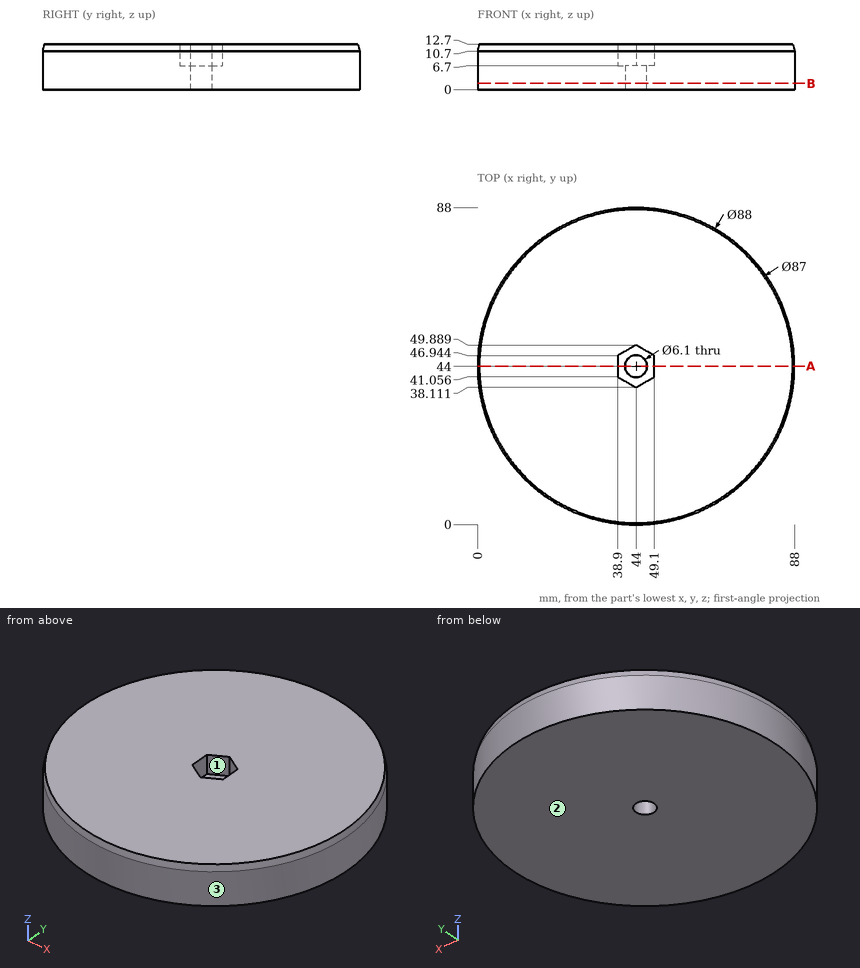
Study the drawing (mm; zero at the part's minimum x, y, z) and answer. Coordinates: 2 decimals unless noted, no trailing zeros. Loops run counter-clockwise (first coordinate to the right, second up) from the corner with the lowest first, then second, coordinate; pieces in that order, holes last. Notation, with made-up numbers: M 81,46.25 L 116,46.25 A13 cw 116,51.25 Z; hole C 45.25,22 d2. An arc over 180 degrees is marked long. Answer in a Markdown table with one row per item.
1) Find section B-B (z = 1.75). Determine the outline of the cut face in (x, y).
Answers below:
| item | result |
|---|---|
| outline | C 44,44 d88; hole C 44,44 d6.1 |
2) Find section A-A (y = 44). Determine the outline of the cut face in (x, z), then the cut area to 3 significant figures.
Answers below:
| item | result |
|---|---|
| outline | M 0,0 L 40.95,0 L 40.95,6.7 L 38.9,6.7 L 38.9,12.7 L 0.5,12.7 L 0,10.7 Z; M 47.05,0 L 88,0 L 88,10.7 L 87.5,12.7 L 49.1,12.7 L 49.1,6.7 L 47.05,6.7 Z |
| area | 1,010 mm^2 |
3) Determine the mould class of the marked faces 1, 2 and 3 for opening direction Y: released by +Y, released by -Y, zero draft, split by the parting line, or undercut.
Answers below:
| item | result |
|---|---|
| face 1 | undercut |
| face 2 | zero draft |
| face 3 | split by the parting line |
4) Given pin 1 (1.5 mm diameter, centred on x = 19, z = 4, fed in from +Y) (1 decimal); pin 2 (1 mm diameter, centred on x = 72.5, z = 10, fed in from +Y); pin 3 (5 mm diameter, centred on y = 55, z = 2.5, fed in from -X), each flat-ended and moving along its own axis, determine where each tip first touches the part or whether it passes through.
Answers below:
| item | result |
|---|---|
| pin 1 | y = 80.7 |
| pin 2 | y = 77.94 |
| pin 3 | x = 0.83 |
5) Find the intervals of material crossed by probe 1 along X at (y, z) = (44, 5.75); probe 2 along Z at (x, y) = (47.5, 47), in increasing order.
Answers below:
| item | result |
|---|---|
| probe 1 | 0 to 40.95, 47.05 to 88 |
| probe 2 | 0 to 6.7 |
